```python
from build123d import *

# Parameters (mm, degrees)
SKETCH1_R                = 6.54812
BOSS_EXTRUDE1_DEPTH      = 1.5
BOSS_EXTRUDE1_DEPTH_BACK = 1.5


with BuildPart() as part:
    # Sketch1 → Boss-Extrude1 (new body, two sides)
    with BuildSketch(Plane(origin=(0, 0, 0), x_dir=(0, 0, -1), z_dir=(1, 0, 0))) as boss_extrude1_sk:
        with BuildLine():
            Line((-12.7, 36.24812), (-12.7, 6.170899448))
            Line((-12.7, 6.170899448), (-11.1, 6.170899448))
            ThreePointArc((-11.1, 6.170899448), (0, 12.7), (11.1, 6.170899448))
            Line((11.1, 6.170899448), (12.7, 6.170899448))
            Line((12.7, 6.170899448), (12.7, 36.24812))
            ThreePointArc((12.7, 36.24812), (0, 48.94812), (-12.7, 36.24812))
        make_face()
        with Locations((0, 36.24812)):
            Circle(SKETCH1_R, mode=Mode.SUBTRACT)
    extrude(amount=BOSS_EXTRUDE1_DEPTH)
    extrude(boss_extrude1_sk.sketch, amount=-BOSS_EXTRUDE1_DEPTH_BACK)


solid = part.part
```
Here's how the part is built. I have some questions about the finished solid (model axes, mm). Round coordinates to 2 decimals unless told otherwise and drop trailing zeros. Loops run counter-clockwise (first coordinate to the right, second up) from the corner with the lowest first, then second, coordinate; pieces in that order, holes last.
1. Thinking about a two-plate mould opening in Y: for faces 1 (the face through (-0.02, 41.77, -3.52)), 2 (the face through (-1.5, 28, 0)), 3 (the face through (0.021, 48.945, -0.279)), 4 (the face through (0, 6.171, -12)), which applies, released by +Y, released by -Y, zero draft, split by the parting line, or undercut?
Answers:
face 1: undercut
face 2: zero draft
face 3: released by +Y
face 4: released by -Y
2. Suppose I cut it at A-A, the plane y = 33. Please give me the cut outline in (x, z), and give its area (3 significant figures).
Answers:
outline: (-1.5, -12.7) - (1.5, -12.7) - (1.5, -5.69) - (-1.5, -5.69) - close; (-1.5, 5.69) - (1.5, 5.69) - (1.5, 12.7) - (-1.5, 12.7) - close
area: 42.1 mm2
3. If I drill on probe 1 along Y at (x, z) = (0.6, 0); probe 2 along Z at (x, y) = (1.4, 40.5); probe 3 along Y at (x, z) = (-0.15, 2.5), over which ranges is the centre line in solid material (lowest first)?
Answers:
probe 1: y = 12.7 to 29.7, 42.8 to 48.95
probe 2: z = -11.97 to -4.98, 4.98 to 11.97
probe 3: y = 12.45 to 30.2, 42.3 to 48.7
4. Suppose I cut it at C-C, the plane x = 0.7. Please give me the cut outline in (y, z).
Answers:
outline: (6.17, -12.7) - (36.25, -12.7) arc R12.7 ccw to (36.25, 12.7) - (6.17, 12.7) - (6.17, 11.1) arc R12.7 cw to (6.17, -11.1) - close; hole circle Ø13.1 at (36.25, 0)
5. Will this pin go through, and if not, where does the flat tip stop? pin 1 (1 mm diameter, centred on x = -0.5, z = 0.5, fed in from -Y).
Answers:
pin 1: stops at y = 12.66
6. Suppose I cut it at B-B, the plane z = 0. Please give me the cut outline in (x, y), and give its area (3 significant figures).
Answers:
outline: (-1.5, 12.7) - (1.5, 12.7) - (1.5, 29.7) - (-1.5, 29.7) - close; (-1.5, 42.8) - (1.5, 42.8) - (1.5, 48.95) - (-1.5, 48.95) - close
area: 69.5 mm2
7. Suppose I cut it at D-D, the plane z = -8.75. Please give me the cut outline in (x, y).
Answers:
outline: (-1.5, 9.2) - (1.5, 9.2) - (1.5, 45.45) - (-1.5, 45.45) - close
